Source: CAD feature listing. Evaluate the final solid. Frame: model axes, mm. A direction names the side the tool comes from. Coordinates: 2 decimals unless noted, no trailing zeros. Loops run counter-clockwise (first coordinate to the right, second up) from the corner with the lowest first, then second, coordinate; pieces in that order, holes last. Notation, with made-up numbers: (25.5, 6) -> (62.5, 6) arc R24 cw to (62.5, 35) -> close; hole circle Ø10 at (-39, 63.25). An arc over 180 degrees is marked (long way). One line per question, with ' | ' between items. Start each with the question number.
```python
from build123d import *

# Parameters (mm, degrees)
F1_DEPTH = 88.9
F3_DEPTH = 6.35
F4_DEPTH = 19.05
F5_R     = 3.175


# Not quite as in the source:
# - a length typed as a fraction of an inch, garbled in the dataset ("3 / 203.2 mm" for 3/8 in), is restored


with BuildPart() as f1:
    # F0 (on Right) → F1 (new body)
    with BuildSketch(Plane.YZ):
        with BuildLine():
            Line((-61.4579357207, 19.05), (-61.4579357207, 66.675))
            Line((-61.4579357207, 66.675), (-70.9829357207, 66.675))
            Line((-70.9829357207, 66.675), (-99.5579357207, 38.1))
            Line((-99.5579357207, 38.1), (-99.5579357207, 31.75))
            Line((-99.5579357207, 31.75), (-112.2579357207, 31.75))
            Line((-112.2579357207, 31.75), (-112.2579357207, 38.1))
            Line((-112.2579357207, 38.1), (-140.8329357207, 66.675))
            Line((-140.8329357207, 66.675), (-150.3579357207, 66.675))
            Line((-150.3579357207, 66.675), (-150.3579357207, 25.4))
            ThreePointArc((-150.3579357207, 25.4), (-152.2178076601, 20.9098719395), (-156.7079357207, 19.05))
            Line((-156.7079357207, 19.05), (-261.4829357207, 19.05))
            Line((-261.4829357207, 19.05), (-261.4829357207, 0))
            Line((-261.4829357207, 0), (-150.3579357207, 0))
            Line((-150.3579357207, 0), (-140.8329357207, 0))
            Line((-140.8329357207, 0), (-74.1579357207, 0))
            Line((-74.1579357207, 0), (-70.9829357207, 0))
            Line((-70.9829357207, 0), (-61.4579357207, 0))
            Line((-61.4579357207, 0), (-61.4579357207, 19.05))
        make_face()
    extrude(amount=-F1_DEPTH)

    # F2 (on face) → F3 (join)
    with BuildSketch(Plane.XY.offset(19.05)):
        with BuildLine():
            Line((-25.4, -228.1454357207), (-25.4, -190.0454357207))
            ThreePointArc((-25.4, -190.0454357207), (-44.45, -170.9954357207), (-63.5, -190.0454357207))
            Line((-63.5, -190.0454357207), (-63.5, -228.1454357207))
            ThreePointArc((-63.5, -228.1454357207), (-44.45, -247.1954357207), (-25.4, -228.1454357207))
        make_face()
        with BuildLine():
            ThreePointArc((-34.925, -228.1454357207), (-44.45, -237.6704357207), (-53.975, -228.1454357207))
            Line((-53.975, -228.1454357207), (-53.975, -190.0454357207))
            ThreePointArc((-53.975, -190.0454357207), (-44.45, -180.5204357207), (-34.925, -190.0454357207))
            Line((-34.925, -190.0454357207), (-34.925, -228.1454357207))
        make_face(mode=Mode.SUBTRACT)
    extrude(amount=F3_DEPTH)

    # F4 (cut): a face of the model
    f4_faces = [f1.faces().sort_by_distance(p)[0] for p in [
        (-44.45, -209.0954357207, 19.05),
    ]]
    extrude(f4_faces, amount=-F4_DEPTH, mode=Mode.SUBTRACT)

    # F5
    f5_edges = [f1.edges().sort_by_distance(p)[0] for p in [
        (-63.5, -209.095436, 19.05),
    ]]
    fillet(f5_edges, radius=F5_R)


solid = f1.part
```
(1) Contact query for flat-ended pins moving along their axis: pin 1 Ø14 at (x, y) = (-56, -108.5) entering from +Z; pin 2 Ø1.6 at (y, z) = (-203.5, 24.5) entering from -X; pin 3 Ø1.5 at (x, y) = (-17.5, -98.5) entering from -Z; pin 4 Ø2 at (x, y) = (-20.5, -96) entering from +Z. Output: stop coordinate, or through.
(2) Cut plane A-A, the plane x = -44.45. Return the cut outline in (y, z) (3 decimals).
(3) Ray query, L1, parallel to Y at x = -59, z = 38; L2, parallel to X at y = -220.5, z = 5 (3 decimals); L3, parallel to Z at x = -13, y = -109. Return the intervals inside material, ascending.
(4) Cut plane B-B, the plane y = -223. Return the cut outline in (x, z) (3 decimals).
(5) Cut plane D-D, the plane y = -161.5. Return the cut outline in (x, z).
(6) Cut plane C-C, the plane x = -11. Return the cut outline in (y, z) (3 decimals).
(7) Access query for faces 5 (the cylindrical face through (-44, -171, 24)), 6 (the flat face through (-44, -99.558, 35)), 7 (the flat face through (-32, -209, 25.4)), 8 (the cylindrical face through (-44.87, -247.19, 23.79)), 9 (the cylindrical face through (-44.659, -180.523, 12.878)). Directions: +Z, -Z, +X, -X, +Y, -Y. A direction counts if a zero-diameter tool reaches every point of the face in a straight line with its end or side. Return the directions, or none.
(8) Draft query along Y for faces 1 (the flat face through (0, -141, 26)), 2 (the flat face through (-44, -261.483, 10)), 3 (the flat face through (-44, -61.458, 33)), 4 (the cylindrical face through (-44.24, -237.67, 12.88)). Return one class per face: pulls with the +Y half, pulls with the -Y half, needs draft (parallel to the pull), parting line crosses it, or undercut.
Here are the results:
1) pin 1: stops at z = 41.34 | pin 2: stops at x = -63.5 | pin 3: stops at z = 0 | pin 4: stops at z = 42.66
2) outline: (-261.483, 0) -> (-237.67, 0) -> (-237.67, 25.4) -> (-247.195, 25.4) -> (-247.195, 22.225) arc R3.175 cw to (-250.37, 19.05) -> (-261.483, 19.05) -> close; (-180.52, 0) -> (-61.458, 0) -> (-61.458, 66.675) -> (-70.983, 66.675) -> (-99.558, 38.1) -> (-99.558, 31.75) -> (-112.258, 31.75) -> (-112.258, 38.1) -> (-140.833, 66.675) -> (-150.358, 66.675) -> (-150.358, 25.4) arc R6.35 cw to (-156.708, 19.05) -> (-167.82, 19.05) arc R3.175 cw to (-170.995, 22.225) -> (-170.995, 25.4) -> (-180.52, 25.4) -> close
3) L1: y = -150.36 to -112.26, -99.56 to -61.46 | L2: x = -88.9 to -53.975, -34.925 to 0 | L3: z = 0 to 31.75
4) outline: (-88.9, 0) -> (-53.975, 0) -> (-53.975, 25.4) -> (-63.5, 25.4) -> (-63.5, 22.225) arc R3.175 cw to (-66.675, 19.05) -> (-88.9, 19.05) -> close; (-34.925, 0) -> (0, 0) -> (0, 19.05) -> (-22.225, 19.05) arc R3.175 cw to (-25.4, 22.225) -> (-25.4, 25.4) -> (-34.925, 25.4) -> close
5) outline: (-88.9, 0) -> (0, 0) -> (0, 19.05) -> (-88.9, 19.05) -> close
6) outline: (-261.483, 0) -> (-61.458, 0) -> (-61.458, 66.675) -> (-70.983, 66.675) -> (-99.558, 38.1) -> (-99.558, 31.75) -> (-112.258, 31.75) -> (-112.258, 38.1) -> (-140.833, 66.675) -> (-150.358, 66.675) -> (-150.358, 25.4) arc R6.35 cw to (-156.708, 19.05) -> (-261.483, 19.05) -> close
7) face 5: +Z | face 6: +Z, +X, -X | face 7: +Z, +X, -X, -Y | face 8: +Z, -Y | face 9: +Z, -Z
8) face 1: needs draft | face 2: pulls with the -Y half | face 3: pulls with the +Y half | face 4: undercut
